```python
from build123d import *

# Parameters (mm, degrees)
SKETCH1_R           = 125.000000063
SKETCH1_R_2         = 6
BOSS_EXTRUDE1_DEPTH = 75
SHELL1_T            = -10
SKETCH2_W           = 14.078706662
SKETCH2_H           = 10.184362198
BOSS_EXTRUDE2_DEPTH = 75
CIRPATTERN1_COUNT   = 21
CUT_EXTRUDE1_REACH  = 841.155
CIRPATTERN2_COUNT   = 7


with BuildPart() as part:
    # Sketch1 → Boss-Extrude1 (new body)
    with BuildSketch(Plane.XY):
        with Locations((-561.018147545, 339.405473748)):
            Circle(SKETCH1_R)
        with Locations((-561.018147545, 339.405473748)):
            Circle(SKETCH1_R_2, mode=Mode.SUBTRACT)
    extrude(amount=BOSS_EXTRUDE1_DEPTH)

    # Shell1
    shell1_openings = [part.faces().sort_by_distance(p)[0] for p in [
        (-682.482613701, 339.405473748, 0),
    ]]
    offset(amount=SHELL1_T, openings=shell1_openings, kind=Kind.INTERSECTION)

    # Sketch2 → Boss-Extrude2 (add)
    with BuildSketch(Plane.XY.offset(75)):
        with Locations((-565.206583335, 464.335282126)):
            Rectangle(SKETCH2_W, SKETCH2_H)
    boss_extrude2 = extrude(amount=-BOSS_EXTRUDE2_DEPTH)

    # CirPattern1: Boss-Extrude2 ×21 about axis
    cirpattern1_axis = Axis((-561.018147545, 339.405473748, 0), (0, 0, 1))
    for i in range(1, CIRPATTERN1_COUNT):
        add(boss_extrude2.rotate(cirpattern1_axis, i * 360 / CIRPATTERN1_COUNT))

    # Sketch3 → Cut-Extrude1 (cut, up to next)
    with BuildSketch(Plane.XY.offset(75), mode=Mode.PRIVATE) as cut_extrude1_sk1:
        with BuildLine():
            Line((-580.05466288, 405.976634587), (-568.983811085, 378.195048585))
            ThreePointArc((-568.983811085, 378.195048585), (-561.018147545, 372.794493792), (-553.052484006, 378.195048585))
            Line((-553.052484006, 378.195048585), (-541.981632211, 405.976634587))
            ThreePointArc((-541.981632211, 405.976634587), (-561.018147545, 434.054949118), (-580.05466288, 405.976634587))
        make_face()
    cut_extrude1_tool1 = extrude(cut_extrude1_sk1.sketch, amount=-CUT_EXTRUDE1_REACH, mode=Mode.PRIVATE) & part.part
    cut_extrude1 = cut_extrude1_tool1.solids().sort_by_distance((-561.018148, 406.56206, 75))[0]
    add(cut_extrude1, mode=Mode.SUBTRACT)

    # CirPattern2: Cut-Extrude1 ×7 about axis
    cirpattern2_axis = Axis((-561.018147545, 339.405473748, 0), (0, 0, 1))
    for i in range(1, CIRPATTERN2_COUNT):
        add(cut_extrude1.rotate(cirpattern2_axis, i * 360 / CIRPATTERN2_COUNT), mode=Mode.SUBTRACT)


solid = part.part
```
Source: CAD feature listing. Evaluate the final solid. Frame: model axes, mm. A direction names the side the tool comes from. Round coordinates to 2 decimals unless told otherwise and drop trailing zeros. Answer as a JSON object with one key per item and string values. Group by question number.
(1) Mould query, pull axis Y, two halves, no side actions, for faces 1 (the flat face through (-500.74, 224.12, 38.02)), 2 (the cylindrical face through (-583.626, 462.344, 36.975)), 3 (the cylindrical face through (-468.874, 317.8, 70.07)). Classes: +Y half, -Y half, draft (parallel to the pull), parting line (faces both ways), or undercut.
(2) Reachability of faces 4 (the cylindrical face through (-685.302, 326.048, 36.975)), 5 (the flat face through (-571.726, 285.875, 70.07)), 6 (the flat face through (-584, 355, 75)) from +Z, -Z, +X, -X, +Y, -Y: full face, straight path, thin tool, end or side. Return the list, or none.
(3) Section query A-A on z = 60. State how many separate pieces and enclosed holes the cut face has, then the cut area to 3 significant figures.
(4) Ray query, line 1 (Y direction, x = -561, z = 50); line 2 (Z direction, x = -626, y = 346.5); line 3 (X direction, y = 309, z = 48). Return the intervals inside material, ascending. Write a range as [from, to].
(5) First-contact query: pin 1 (5 mm diameter, centred on y = 385, z = 37.5, fed in from -X); pin 2 (6 mm diameter, centred on x = -483.5, z = 40, fed in from +Y); pin 3 (12 mm diameter, centred on x = -489, y = 284.5, fed in from -Z); pin 4 (6 mm diameter, centred on x = -597.5, y = 379, fed in from -Z). Flat tips, straight axial feed; report the tip coordinate or a pass-through.
Computed values:
{
 "1": {"face 1": "-Y half", "face 2": "+Y half", "face 3": "undercut"},
 "2": {"face 4": "+Z, -Z, -X", "face 5": "+Z, -Z", "face 6": "+Z, +X, -X, +Y, -Y"},
 "3": {"separate pieces": "2", "enclosed holes": "2", "area": "9,760 mm^2"},
 "4": {"line 1": "[214.41, 224.41], [323.41, 333.41], [345.41, 355.41], [454.41, 469.43]", "line 2": "[65, 75]", "line 3": "[-687.44, -671.93], [-450.11, -434.59]"},
 "5": {"pin 1": "x = -683.78", "pin 2": "y = 445.97", "pin 3": "z = 65", "pin 4": "through"}
}
